Autodesk Inventor part; units mm, degrees
ref_plane "YZ Plane" through (0, 0, 0) normal (1, 0, 0) x (0, 1, 0)
ref_plane "XZ Plane" through (0, 0, 0) normal (0, 1, 0) x (-1, 0, 0)
ref_plane "XY Plane" through (0, 0, 0) normal (0, 0, 1) x (1, 0, 0)
sketch "Sketch1" plane through (0, 0, 0) normal (0, 0, 1) x (1, 0, 0)
  circle A0 centre (11, 6) radius 2.7 construction
  circle A1 centre (11, -6) radius 2.7 construction
  line L0 (49.7615, -342.4426) -> (49.7615, 314.6303) construction
  line L1 (11, 12) -> (-4.4335, 12) construction
  line L2 (-17, -12) -> (11, -12) construction
  line L3 (4, 12) -> (4, -12)
  line L4 (4, 12) -> (11, 19)
  line L5 (11, 19) -> (49.7615, 19)
  line L6 (19.0192, 2.5843) -> (28.2364, 13.6384) construction
  circle A2 centre (11, 6) radius 3
  circle A3 centre (11, -6) radius 3
  circle A4 centre (88.5231, 6) radius 3
  circle A5 centre (88.5231, -6) radius 3
  line L7 (4, -12) -> (29.7615, -31)
  line L8 (29.7615, -31) -> (49.7615, -31)
  line L9 (95.5231, 12) -> (95.5231, -12)
  line L10 (95.5231, 12) -> (88.5231, 19)
  line L11 (88.5231, 19) -> (49.7615, 19)
  line L12 (95.5231, -12) -> (69.7615, -31)
  line L13 (69.7615, -31) -> (49.7615, -31)
  point P0 (0, 0)
  dimension "d0" = 7
  dimension "d6" = 6
  dimension "d7" = 6
  dimension "d14" = 7
  dimension "d15" = 50
  dimension "d16" = 20
  dimension "d38" = 135
extrude "Plate1" add sketch "Sketch1" along normal blind 3
sketch "Sketch5" plane through (0, 0, 3) normal (0, 0, 1) x (1, 0, 0)
  circle A0 centre (88.5231, -6) radius 3 construction
  line L0 (4, -12) -> (4, 12) construction
  line L1 (29.7615, -31) -> (4, -12) construction
  line L2 (69.7615, -31) -> (29.7615, -31) construction
  line L3 (95.5231, -12) -> (69.7615, -31) construction
  line L4 (95.5231, 12) -> (95.5231, -12) construction
  line L5 (88.5231, 19) -> (95.5231, 12) construction
  line L6 (11, 19) -> (88.5231, 19) construction
  line L7 (4, 12) -> (11, 19) construction
  line L8 (85.2094, 11) -> (87.5231, 8.6863) construction
  line L9 (87.5231, 8.6863) -> (87.5231, -7.9598) construction
  line L10 (87.5231, -7.9598) -> (67.1305, -23) construction
  line L11 (67.1305, -23) -> (32.3926, -23) construction
  line L12 (32.3926, -23) -> (12, -7.9598) construction
  line L13 (12, -7.9598) -> (12, 8.6863) construction
  line L14 (12, 8.6863) -> (14.3137, 11) construction
  line L15 (14.3137, 11) -> (85.2094, 11) construction
  line L16 (18, 11) -> (18, -12.385) construction
  line L17 (49.7615, 11) -> (49.7615, -23) construction
  line L18 (81.5231, 11) -> (81.5231, -12.385) construction
  line L19 (33.6401, 11) -> (19.5, -13.4913) construction
  line L20 (29.542, 9.9019) -> (18.4019, -9.3932)
  line L21 (23.5981, -12.3932) -> (34.7381, 6.9019)
  arc A1 (34.7381, 6.9019) -> (29.542, 9.9019) centre (32.1401, 8.4019) ccw
  arc A2 (18.4019, -9.3932) -> (23.5981, -12.3932) centre (21, -10.8932) ccw
  line L22 (45.1871, 11) -> (27.5985, -19.4642) construction
  line L23 (41.089, 9.9019) -> (26.5005, -15.3662)
  line L24 (31.6966, -18.3662) -> (46.2851, 6.9019)
  arc A3 (46.2851, 6.9019) -> (41.089, 9.9019) centre (43.6871, 8.4019) ccw
  arc A4 (26.5005, -15.3662) -> (31.6966, -18.3662) centre (29.0985, -16.8662) ccw
  line L25 (56.7341, 11) -> (37.1042, -23) construction
  line L26 (52.636, 9.9019) -> (36.0061, -18.9019)
  line L27 (41.2022, -21.9019) -> (57.8321, 6.9019)
  arc A5 (57.8321, 6.9019) -> (52.636, 9.9019) centre (55.2341, 8.4019) ccw
  arc A6 (36.0061, -18.9019) -> (41.2022, -21.9019) centre (38.6042, -20.4019) ccw
  line L28 (68.2811, 11) -> (48.6512, -23) construction
  line L29 (64.183, 9.9019) -> (47.5531, -18.9019)
  line L30 (52.7492, -21.9019) -> (69.3791, 6.9019)
  arc A7 (69.3791, 6.9019) -> (64.183, 9.9019) centre (66.7811, 8.4019) ccw
  arc A8 (47.5531, -18.9019) -> (52.7492, -21.9019) centre (50.1512, -20.4019) ccw
  line L31 (79.8281, 11) -> (60.1982, -23) construction
  line L32 (75.73, 9.9019) -> (59.1001, -18.9019)
  line L33 (64.2962, -21.9019) -> (80.9262, 6.9019)
  arc A9 (80.9262, 6.9019) -> (75.73, 9.9019) centre (78.3281, 8.4019) ccw
  arc A10 (59.1001, -18.9019) -> (64.2962, -21.9019) centre (61.6982, -20.4019) ccw
  point P0 (26.57, -1.2456)
  point P1 (36.3928, -4.2321)
  point P2 (46.9191, -6)
  point P3 (58.4661, -6)
  point P4 (70.0131, -6)
  dimension "d61" = 8
  dimension "d62" = 14
  dimension "d63" = 3
  dimension "d64" = 60
  dimension "d65" = 4
  dimension "d66" = 4
  dimension "d67" = 4
  dimension "d68" = 4
extrude "Cut2" cut sketch "Sketch5" against normal blind 3
equation "\"d9\" = Thickness"
equation "\"BendRadius\" = Thickness"
equation "\"BendReliefWidth\" = Thickness"
equation "\"BendReliefDepth\" = 0.5 * Thickness"
equation "\"CornerReliefSize\" = 4 * Thickness"
equation "\"MinimumRemnant\" = 2 * Thickness"
equation "\"TransitionRadius\" = BendRadius"
equation "\"JacobiRadiusSize\" = BendRadius"
equation "\"GapSize\" = Thickness"
properties part number "NoseMount"
Input: part model. Units: mm. Frame: model coordinates. A direction names the side the tool comes from. Give positions to 0.01 mm unless a question says otherwise; leave off trailing zeros. Order: outer loops, then holes, each group sorted by start corner. A loop starts at its lowest first (then second) coordinate and runs counter-clockwise, first axis right, second up. Notation, with made-up numbers: M 56,-14 L 70,-14 A25 cw 70,5 Z; hole C -34,59 d10. An arc over 180 degrees is marked long. Return JSON: item names as keys, results as strings.
Item 1: Cut plane B-B (x = 79). Return loops of the section in (y, z), then the cut area to 3 significant figures.
Solutions:
{"outline": "M -24.19,0 L 3.57,0 L 3.57,3 L -24.19,3 Z; M 11.33,0 L 19,0 L 19,3 L 11.33,3 Z", "area": "106 mm^2"}
Item 2: Pull-direction query (X, two-part tool) for faces 1 (the flat face through (49, 19, 1)), 2 (the flat face through (49.4, -7.7, 1.5)), 3 (the flat face through (16.7, -21.367, 1.479)); classes: +X half, -X half, draft (parallel to the pull), parting line (faces both ways), or undercut.
Solutions:
{"face 1": "draft", "face 2": "undercut", "face 3": "-X half"}
Item 3: Cut plane C-C (x = 66.5). Return loops of the section in (y, z), then the cut area to 3 significant figures.
Solutions:
{"outline": "M -31,0 L -18.08,0 L -18.08,3 L -31,3 Z; M -6.08,0 L 1.92,0 L 1.92,3 L -6.08,3 Z; M 11.39,0 L 19,0 L 19,3 L 11.39,3 Z", "area": "85.6 mm^2"}
Item 4: Access query for faces 4 (the flat face through (29.09, -2.88, 1.52)), 5 (the flat face through (49, -11, 0)). Directions: +Z, -Z, +X, -X, +Y, -Y. A direction counts if a zero-diameter tool reaches every point of the face in a straight line with its end or side. Return the directions, or none.
Solutions:
{"face 4": "+Z, -Z", "face 5": "-Z, +X, -X, +Y, -Y"}
Item 5: Ray query, probe 1 along Y at (x, z) = (11, 2.15); probe 2 along Y at (x, z) = (88, 0.65); probe 3 along X at (y, z) = (-19, 1.5). Return the intervals inside material, ascending.
Solutions:
{"probe 1": "-17.16 to -9, -3 to 3, 9 to 19", "probe 2": "-17.55 to -8.95, -3.05 to 3.05, 8.95 to 19", "probe 3": "13.49 to 26.99, 31.21 to 35.95, 42.88 to 47.5, 54.42 to 59.05, 65.97 to 86.03"}
Item 6: Cut plane A-A (z = 2.4). State how many separate pieces and enclosed holes the cut face has, then the cut area to 3 significant figures.
Solutions:
{"separate pieces": "1", "enclosed holes": "9", "area": "2,880 mm^2"}
